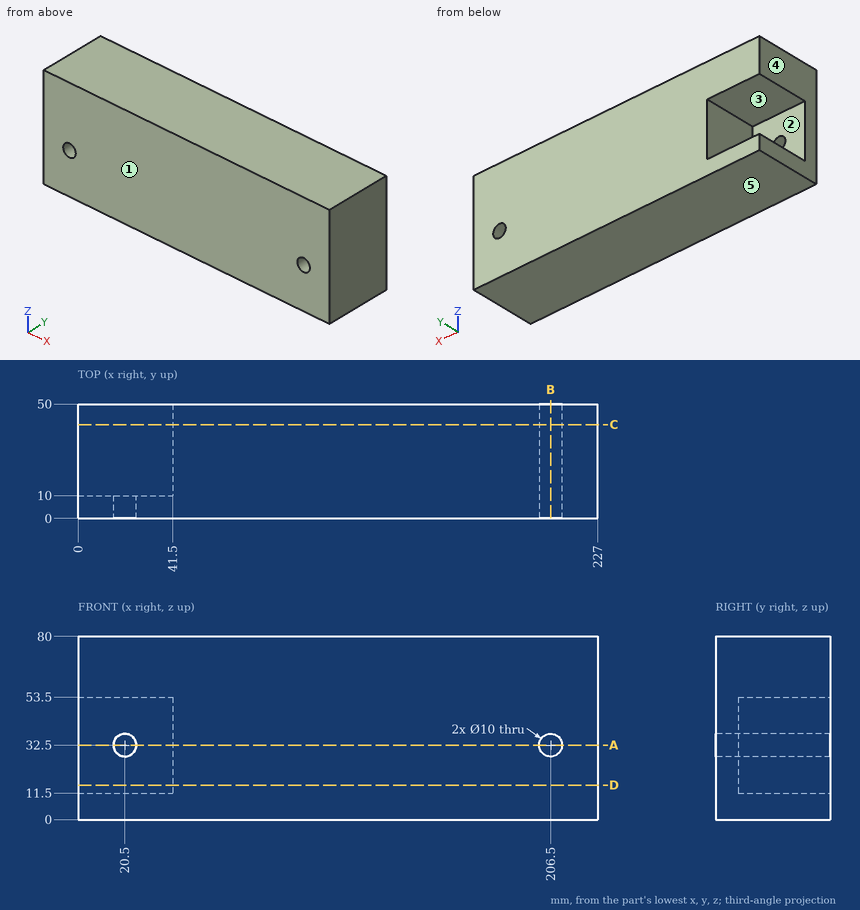
Could you check a few things on this drawing? It's one solid part, dimensions in mm from its lowest x, y, z. A direction names the side the tool comes from. Coordinates: 2 decimals unless noted, no trailing zeros. Order: outer loops, then holes, each group sorted by start corner. A loop starts at its lowest first (then second) coordinate and runs counter-clockwise, first axis right, second up. Notation, with made-up numbers: (-23.5, 13.25) - (17.5, 13.25) arc R21 cw to (17.5, 44.25) - close; hole circle Ø2 at (-28.75, -17). An arc over 180 degrees is marked (long way). One line per question, with ' | ' between items. Start each with the question number.
1. If we mould it in two halves opening along Z, with no side actions, what happens to the marked faces 3, 4 and 5? For each: released by +Z, released by -Z, zero draft, split by the parting line, or undercut.
2. If we section it at C-C (y = 41): Write out the boundary of the cut face in (x, z).
3. If we section it at B-B (x = 206.5): Write out the boundary of the cut face in (y, z).
4. Please list where these lines run through material, in increasing order: line 1 along X through (y, z) = (4, 32); line 2 along Z through (x, y) = (206.5, 35); line 3 along Z through (x, y) = (18, 32.5). Write a range as [from, to].
5. Which directions (+Z, -Z, +X, -X, +Y, -Y) give clear straight access to the entire face, cutting with the end or side of a thin tool? Please do the marked faces 1 and 2.
6. If we section it at D-D (z = 15): Write out the boundary of the cut face in (x, y), and give its area (3 significant figures).
7. If we section it at A-A (z = 32.5): Write out the boundary of the cut face in (x, y), and give its area (3 significant figures).
8. I'm going to push flat-ended pins straight in: pin 1 Ø10 at (x, y) = (124, 30) entering from -Z; pin 2 Ø2 at (y, z) = (22.5, 18) entering from -X. Where does each tip first touch, or does it pass through?
Model answer:
1) face 3: undercut | face 4: zero draft | face 5: released by -Z
2) outline: (0, 0) - (227, 0) - (227, 80) - (0, 80) - (0, 53.5) - (41.5, 53.5) - (41.5, 11.5) - (0, 11.5) - close; hole circle Ø10 at (206.5, 32.5)
3) outline: (0, 0) - (50, 0) - (50, 27.5) - (0, 27.5) - close; (0, 37.5) - (50, 37.5) - (50, 80) - (0, 80) - close
4) line 1: x = [0, 15.53], [25.47, 201.53], [211.47, 227] | line 2: z = [0, 27.5], [37.5, 80] | line 3: z = [0, 11.5], [53.5, 80]
5) face 1: +Z, -Z, +X, -X, -Y | face 2: -X, +Y
6) outline: (0, 0) - (227, 0) - (227, 50) - (41.5, 50) - (41.5, 10) - (0, 10) - close | area: 9,690 mm²
7) outline: (0, 0) - (15.5, 0) - (15.5, 10) - (0, 10) - close; (25.5, 0) - (201.5, 0) - (201.5, 50) - (41.5, 50) - (41.5, 10) - (25.5, 10) - close; (211.5, 0) - (227, 0) - (227, 50) - (211.5, 50) - close | area: 9,090 mm²
8) pin 1: stops at z = 0 | pin 2: stops at x = 41.5
